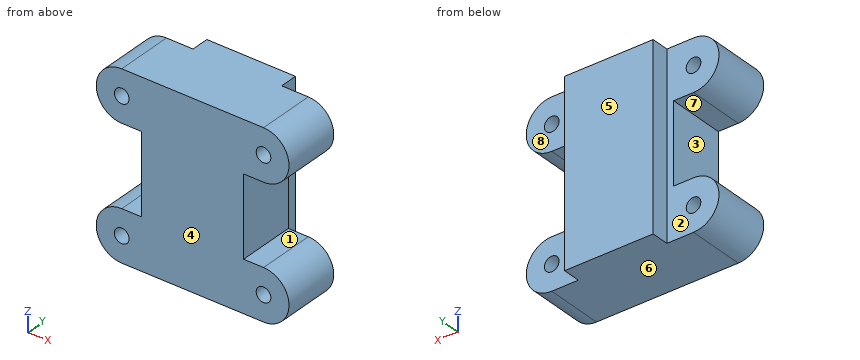
from build123d import *

# Parameters (mm, degrees)
SKETCH1_R           = 1.65
BOSS_EXTRUDE1_DEPTH = 13
SKETCH2_W           = 20
SKETCH2_H           = 41
BOSS_EXTRUDE2_DEPTH = 4


with BuildPart() as part:
    # Sketch1 → Boss-Extrude1 (new body)
    with BuildSketch(Plane(origin=(0, 0, 0), x_dir=(1, 0, 0), z_dir=(0, 1, 0))):
        with BuildLine():
            Line((-16, 9), (-11.5, 9))
            Line((-11.5, 9), (-11.5, -9))
            Line((-11.5, -9), (-16, -9))
            ThreePointArc((-16, -9), (-21.75, -14.75), (-16, -20.5))
            Line((-16, -20.5), (16, -20.5))
            ThreePointArc((16, -20.5), (21.75, -14.75), (16, -9))
            Line((16, -9), (11.5, -9))
            Line((11.5, -9), (11.5, 9))
            Line((11.5, 9), (16, 9))
            ThreePointArc((16, 9), (21.75, 14.75), (16, 20.5))
            Line((16, 20.5), (-16, 20.5))
            ThreePointArc((-16, 20.5), (-21.75, 14.75), (-16, 9))
        make_face()
        with Locations(Location((-16, 14.75, 0), (0, 0, 90))):
            Circle(SKETCH1_R, mode=Mode.SUBTRACT)
        with Locations(Location((16, 14.75, 0), (0, 0, 90))):
            Circle(SKETCH1_R, mode=Mode.SUBTRACT)
        with Locations(Location((16, -14.75, 0), (0, 0, 90))):
            Circle(SKETCH1_R, mode=Mode.SUBTRACT)
        with Locations(Location((-16, -14.75, 0), (0, 0, 90))):
            Circle(SKETCH1_R, mode=Mode.SUBTRACT)
    extrude(amount=BOSS_EXTRUDE1_DEPTH)

    # Sketch2 → Boss-Extrude2 (add)
    with BuildSketch(Plane(origin=(0, 13, 0), x_dir=(1, 0, 0), z_dir=(0, 1, 0))):
        Rectangle(SKETCH2_W, SKETCH2_H)
    extrude(amount=BOSS_EXTRUDE2_DEPTH)


solid = part.part
Geometry: final body of the model. Coordinates: model frame, mm. Face numbers are marked on the shaded views. A direction names the side the tool comes from. Round coordinates to 2 decimals unless told otherwise and drop trailing zeros. Loops run counter-clockwise (first coordinate to the right, second up) from the corner with the lowest first, then second, coordinate; pieces in that order, holes last. Notation, with made-up numbers: M -1.75,-8 L 42.25,-8 A13 cw 42.25,13 Z; hole C 50.5,28 d9. An arc over 180 degrees is marked long. One line per question, with ' | ' between items.
(1) Pull-direction query (Z, two-part tool) for the marked faces 6, 7 and 8; classes: +Z half, -Z half, draft (parallel to the pull), parting line (faces both ways), or undercut.
Check result:
face 6: -Z half | face 7: undercut | face 8: draft
(2) Contact query for flat-ended pins moving along their axis: P1, Ø6, axis at x = -17, y = 9.5, coming from the -Z side; P2, Ø3, axis at x = 16, z = 14.75, coming from the +Y side; P3, Ø5, axis at y = 7, z = -1.5, coming from the +X side; P4, Ø6, axis at y = 2.5, z = 3, coming from the -X side. Output: stop coordinate, or through.
Check result:
P1: stops at z = -20.5 | P2: passes through | P3: stops at x = 11.5 | P4: stops at x = -11.5
(3) Cut plane B-B on z = -14.75. Return the cut outline in (x, y), plus the area to 3 significant figures.
Check result:
outline: M -21.75,0 L -17.65,0 L -17.65,13 L -21.75,13 Z; M -14.35,0 L 14.35,0 L 14.35,13 L 10,13 L 10,17 L -10,17 L -10,13 L -14.35,13 Z; M 17.65,0 L 21.75,0 L 21.75,13 L 17.65,13 Z | area: 560 mm2
(4) Cut plane A-A on y = 7. Return the cut outline in (x, z), plus the area to 3 significant figures.
Check result:
outline: M -16,-20.5 L 16,-20.5 A5.75 ccw 16,-9 L 11.5,-9 L 11.5,9 L 16,9 A5.75 ccw 16,20.5 L -16,20.5 A5.75 ccw -16,9 L -11.5,9 L -11.5,-9 L -16,-9 A5.75 ccw Z; hole C -16,-14.75 d3.3; hole C -16,14.75 d3.3; hole C 16,-14.75 d3.3; hole C 16,14.75 d3.3 | area: 1,320 mm2
(5) Cut plane C-C on x = -17. Return the cut outline in (y, z), plus the area to 3 significant figures.
Check result:
outline: M 0,-20.41 L 13,-20.41 L 13,-16.06 L 0,-16.06 Z; M 0,-13.44 L 13,-13.44 L 13,-9.09 L 0,-9.09 Z; M 0,9.09 L 13,9.09 L 13,13.44 L 0,13.44 Z; M 0,16.06 L 13,16.06 L 13,20.41 L 0,20.41 Z | area: 226 mm2
(6) Access query for the marked faces 1, 2, 3, 4 and 5. Directions: +Z, -Z, +X, -X, +Y, -Y. A direction counts if a zero-diameter tool reaches every point of the face in a straight line with its end or side. Return the directions, or none.
Check result:
face 1: +X, +Y, -Y | face 2: +Z, -Z, -X, +Y | face 3: -X, +Y, -Y | face 4: +Z, -Z, +X, -X, -Y | face 5: +Z, -Z, +X, -X, +Y
(7) Material intervals for line 1 along X through (y, z) = (5.25, 14.75); line 2 along Z through (x, y) = (16, 9); line 3 along X through (y, z) = (2.25, -2.5), sorted ascending. Write a range as from..to.
Check result:
line 1: x = -21.75..-17.65, -14.35..14.35, 17.65..21.75 | line 2: z = -20.5..-16.4, -13.1..-9, 9..13.1, 16.4..20.5 | line 3: x = -11.5..11.5
(8) Cut plane D-D on z = 7. Return the cut outline in (x, y).
Check result:
outline: M -11.5,0 L 11.5,0 L 11.5,13 L 10,13 L 10,17 L -10,17 L -10,13 L -11.5,13 Z
